from build123d import *

# Parameters (mm, degrees)
F0_W     = 13
F0_H     = 20
F0_R     = 4
F0_W_2   = 6
F0_H_2   = 3.5
F1_DEPTH = 6
F2_DEPTH = 0.5
F3_R     = 4
F4_DEPTH = 27
F5_R     = 2
F7_DEPTH = 20
F8_R     = 5
F9_R     = 2.99999


# Not quite as in the source:
# - a fillet or chamfer is up to 0.001 mm smaller than in the source, because OpenCascade refuses the exact size


with BuildPart() as f1:
    # F0 (on Top) → F1 (new body)
    with BuildSketch(Plane.XY):
        Polygon((25, 75), (-25, 75), (-25, 22), (0, 22), (25, 22), align=None)
        Polygon((-21, 28.5), (-21, 65), (-15, 65), (-15, 28.5), (-15, 25), (-21, 25), align=None, mode=Mode.SUBTRACT)
        with BuildLine():
            ThreePointArc((5, 27), (3.5355339059, 23.4644660941), (0, 22))
            ThreePointArc((0, 22), (-3.5355339059, 30.5355339059), (5, 27))
        make_face(mode=Mode.SUBTRACT)
        with Locations((0, 45)):
            Rectangle(F0_W, F0_H, mode=Mode.SUBTRACT)
        Polygon((21, 25), (15, 25), (15, 28.5), (15, 65), (21, 65), (21, 28.5), align=None, mode=Mode.SUBTRACT)
        with BuildLine():
            ThreePointArc((5, 27), (-3.5355339059, 30.5355339059), (0, 22))
            ThreePointArc((0, 22), (3.5355339059, 23.4644660941), (5, 27))
        make_face()
        with Locations((0, 27)):
            Circle(F0_R, mode=Mode.SUBTRACT)
        with Locations((0, 27)):
            Circle(F0_R)
        with Locations((18, 26.75)):
            Rectangle(F0_W_2, F0_H_2)
        with Locations((-18, 26.75)):
            Rectangle(F0_W_2, F0_H_2)
    extrude(amount=-F1_DEPTH)

    # F0 (on Top) → F2 (join)
    with BuildSketch(Plane.XY):
        with BuildLine():
            ThreePointArc((5, 27), (-3.5355339059, 30.5355339059), (0, 22))
            ThreePointArc((0, 22), (3.5355339059, 23.4644660941), (5, 27))
        make_face()
        with Locations((0, 27)):
            Circle(F0_R, mode=Mode.SUBTRACT)
        with Locations((0, 27)):
            Circle(F0_R)
    extrude(amount=F2_DEPTH)

    # F3 (on face) → F4 (join)
    with BuildSketch(Plane.XY.offset(0.5)):
        with Locations((0, 27)):
            Circle(F3_R)
    extrude(amount=F4_DEPTH)

    # F5
    f5_edges = [f1.edges().sort_by_distance(p)[0] for p in [
        (-4, 27, 27.5),
    ]]
    fillet(f5_edges, radius=F5_R)

    # F6 (on face) → F7 (cut, through all)
    with BuildSketch(Plane(origin=(0, 75, 0), x_dir=(-1, 0, 0), z_dir=(0, 1, 0))):
        with BuildLine():
            ThreePointArc((-1.5, -3), (0, -4.5), (1.5, -3))
            ThreePointArc((1.5, -3), (0, -1.5), (-1.5, -3))
        make_face()
        with BuildLine():
            ThreePointArc((-1.5, -3), (0, -1.5), (1.5, -3))
            Line((1.5, -3), (1.5, 0))
            Line((1.5, 0), (-1.5, 0))
            Line((-1.5, 0), (-1.5, -3))
        make_face()
    extrude(amount=-F7_DEPTH, mode=Mode.SUBTRACT)

    # F8
    f8_edges = [f1.edges().sort_by_distance(p)[0] for p in [
        (25, 75, -3),
        (-25, 75, -3),
        (-25, 22, -3),
        (25, 22, -3),
    ]]
    fillet(f8_edges, radius=F8_R)

    # F9 (radius 3 in the source; OpenCascade refuses exactly that, so slightly less here)
    f9_edges = [f1.edges().sort_by_distance(p)[0] for p in [
        (-15, 28.5, -3),
        (-21, 28.5, -3),
        (21, 28.5, -3),
        (15, 28.5, -3),
        (21, 65, -3),
        (-15, 65, -3),
        (-21, 65, -3),
        (15, 65, -3),
    ]]
    fillet(f9_edges, radius=F9_R)


solid = f1.part
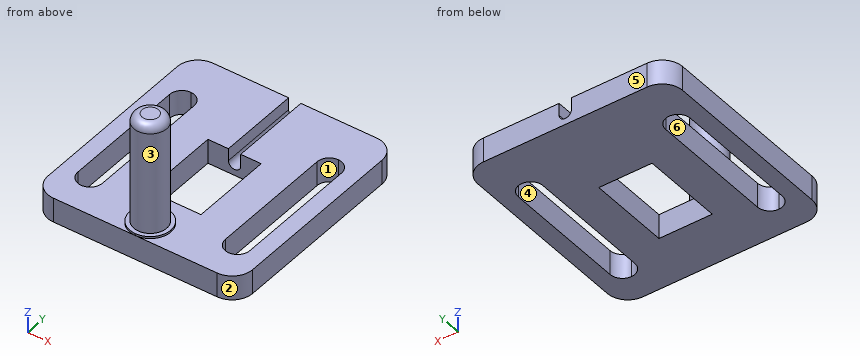
Build history of the part. All positions in model axes, mm. Face numbers are marked on the shaded views. A direction names the side the tool comes from. Coordinates: 2 decimals unless noted, no trailing zeros. Order: outer loops, then holes, each group sorted by start corner. A loop starts at its lowest first (then second) coordinate and runs counter-clockwise, first axis right, second up. Notation, with made-up numbers: (85, 33.25) - (95, 33.25) arc R25 cw to (95, 67.25) - close; hole circle Ø1 at (-22.75, 49.25). An arc over 180 degrees is marked (long way). Write item = value, one per line. Start each with the question number.
1) Saw through at C-C on y = 57. Write the cut outline in (x, z).
2) Wall check: line 1 along X through (y, z) = (49.5, -3); line 2 along Z through (x, y) = (13, 27); line 3 along Z through (x, y) = (1, 56). Give the ranges that are in metal, low to high. Write a range as from..to.
3) Flat gauge pins, fed straight in: pin 1 Ø12 at (x, z) = (1, 12.5) entering from +Y; pin 2 Ø15 at (x, y) = (-5.5, 48.5) entering from +Z. Where does each tip first touch, or does it go through?
4) Saw through at B-B on z = -1. Count the separate pieces of the cut face and the enclosed holes in it, then the cut area to 3 significant figures.
5) Saw through at A-A on y = 43. Write the cut outline in (x, z), then the cut area to 3 significant figures.
6) 3-axis set-ups, long thin cutter, end or side, ignore diameter. For the marked faces 1 and 2: which of +Z, -Z, +X, -X, +Y, -Y reach the whole face in a straight line?
7) Saw through at D-D on x = -19. Write the cut outline in (y, z), then the cut area to 3 significant figures.
8) Two-plate mould, pull along Y, no slides. Class the marked faces 3, 4, 5 and 6: pulls with the +Y half, pulls with the -Y half, needs draft (parallel to the pull), parting line crosses it, or undercut.
From the geometry:
q1.outline = (-25, -6) - (-21, -6) - (-21, 0) - (-25, 0) - close; (-15, -6) - (15, -6) - (15, 0) - (1.5, 0) - (1.5, -3) arc R1.5 cw to (-1.5, -3) - (-1.5, 0) - (-15, 0) - close; (21, -6) - (25, -6) - (25, 0) - (21, 0) - close
q2.line_1 = -25..-21, -15..-6.5, 6.5..15, 21..25
q2.line_2 = -6..0
q2.line_3 = -6..-4.12
q3.pin_1 = 31
q3.pin_2 = 0
q4.separate_pieces = 1
q4.enclosed_holes = 2
q4.area = 1,890 mm^2
q5.outline = (-25, -6) - (-21, -6) - (-21, 0) - (-25, 0) - close; (-15, -6) - (-6.5, -6) - (-6.5, 0) - (-15, 0) - close; (6.5, -6) - (15, -6) - (15, 0) - (6.5, 0) - close; (21, -6) - (25, -6) - (25, 0) - (21, 0) - close
q5.area = 150 mm^2
q6.face_1 = +Z, -Z
q6.face_2 = +Z, -Z, +X, -Y
q7.outline = (22, -6) - (28.67, -6) - (28.67, 0) - (22, 0) - close; (64.83, -6) - (75, -6) - (75, 0) - (64.83, 0) - close
q7.area = 101 mm^2
q8.face_3 = parting line crosses it
q8.face_4 = undercut
q8.face_5 = pulls with the +Y half
q8.face_6 = undercut
